from build123d import *

# Parameters (mm, degrees)
F0_W = 19.261638
F0_H = 2.626098


with BuildPart() as f1:
    # F0 (on Front) → F1 (revolve)
    with BuildSketch(Plane.XZ):
        with Locations((11.864158, 1.313049)):
            Rectangle(F0_W, F0_H)
        Polygon((21.092495, 0.527442), (2.693319, 0.498693), (2.693319, 2.223616), (21.092495, 2.223616), align=None, mode=Mode.SUBTRACT)
    revolve(axis=Axis((2.233339, 0, 1.313049), (0, 0, 1)))


solid = f1.part
Read the model definition and answer for the solid it produces. Units are mm, in the model's axes. A direction names the side the tool comes from. Give positions to 0.01 mm unless a question says otherwise; leave off trailing zeros. Loops run counter-clockwise (first coordinate to the right, second up) from the corner with the lowest first, then second, coordinate; pieces in that order, holes last. Notation, with made-up numbers: M 44.25,72.5 L 68.25,72.5 A19 cw 68.25,76.5 Z; hole C -27.75,27.5 d8. An arc over 180 degrees is marked long. Write each question's results on one line, items separated by ' | '.
1. Straight lines are drawn through the part: line 1 (Z direction, x = 4.5, y = -7); line 2 (X direction, y = -3, z = 2.1); line 3 (Y direction, x = 15.5, z = 1.45). For each, find the intervals that lie inside material, in ascending order. Write a range as [from, to].
Values:
line 1: z = [0, 0.51], [2.22, 2.63] | line 2: x = [-16.79, -16.39], [20.85, 21.26] | line 3: y = [-13.96, -13.4], [13.4, 13.96]
2. Section B-B on y = 0 is taken. Give the vertices of the cut face in (x, z).
Values:
outline: M -17.03,0 L 21.49,0 L 21.49,2.63 L -17.03,2.63 Z; hole M -16.63,0.53 L 1.77,0.5 L 1.77,2.22 L -16.63,2.22 Z; hole M 2.69,0.5 L 21.09,0.53 L 21.09,2.22 L 2.69,2.22 Z
3. The mould has two halves that part along Z. Classify faces 3 (the face through (2.67, 0.14, 1.37)), 4 (the face through (11.1, -17.1, 1.3)), 5 (the face through (3, 0, 2.626)): pulls with the +Z half, pulls with the -Z half, needs draft (parallel to the pull), parting line crosses it, or undercut.
Values:
face 3: undercut | face 4: needs draft | face 5: pulls with the +Z half
4. Given pin 1 (1 mm diameter, centred on y = -9, z = 1, fed in from -X); pin 2 (1 mm diameter, centred on x = -7, z = 1.5, fed in from +Y), each flat-ended and moving along its own axis, determine where each tip first touches the part or whether it passes through.
Values:
pin 1: stops at x = -15.05 | pin 2: stops at y = 17.17
5. A tool of negligible diameter and unlimited length cuts with its end or side. For faces 1 (the face through (-12.73, -11.48, 1.36)), 2 (the face through (3, 0, 0)), from which of +Z, -Z, +X, -X, +Y, -Y can it reach the whole face along a straight path? Write none if from no direction.
Values:
face 1: none | face 2: -Z, +X, -X, +Y, -Y
6. Section A-A on z = 1.2 is taken. Give the vertices of the cut face in (x, y), plus the area to 3 significant figures.
Values:
outline: C 2.23,0 d38.52; C 2.23,0 d0.92; hole C 2.23,0 d37.72 | area: 48.9 mm^2
